```python
from build123d import *

# Parameters (mm, degrees)
F1_DEPTH = 88.9
F2_START = 25.4
F2_DEPTH = 19.05


with BuildPart() as f1:
    # F0 (on Front) → F1 (new body)
    with BuildSketch(Plane.XZ):
        Polygon((-284.0362622675, 569.4989632036), (-303.0862622675, 588.5489632036), (-303.0862622675, -313.1510367964), (-284.0362622675, -294.1010367964), align=None)
        Polygon((243.0137377325, 588.5489632036), (-303.0862622675, 588.5489632036), (-284.0362622675, 569.4989632036), (223.9637377325, 569.4989632036), align=None)
        Polygon((-284.0362622675, -294.1010367964), (-303.0862622675, -313.1510367964), (243.0137377325, -313.1510367964), (223.9637377325, -294.1010367964), align=None)
        Polygon((243.0137377325, -313.1510367964), (243.0137377325, 588.5489632036), (223.9637377325, 569.4989632036), (223.9637377325, -294.1010367964), align=None)
    extrude(amount=F1_DEPTH)

    # F0 (on Front) → F2 (join)
    with BuildSketch(Plane.XZ.offset(F2_START)):
        Polygon((223.9637377325, 569.4989632036), (-284.0362622675, 569.4989632036), (-245.9362622675, 531.3989632036), (185.8637377325, 531.3989632036), align=None)
        Polygon((-245.9362622675, 531.3989632036), (-284.0362622675, 569.4989632036), (-284.0362622675, -294.1010367964), (-245.9362622675, -256.0010367964), align=None)
        Polygon((223.9637377325, -294.1010367964), (223.9637377325, 569.4989632036), (185.8637377325, 531.3989632036), (185.8637377325, -256.0010367964), align=None)
        Polygon((-245.9362622675, -256.0010367964), (-284.0362622675, -294.1010367964), (223.9637377325, -294.1010367964), (185.8637377325, -256.0010367964), align=None)
    extrude(amount=F2_DEPTH)


solid = f1.part
```
Model file for the job. Use its own axes, mm. A direction names the side the tool comes from. Coordinates: 2 decimals unless noted, no trailing zeros. Order: outer loops, then holes, each group sorted by start corner. A loop starts at its lowest first (then second) coordinate and runs counter-clockwise, first axis right, second up. Notation, with made-up numbers: (49.25, -36.75) -> (80.25, -36.75) arc R30 ccw to (80.25, 2.25) -> close; hole circle Ø6 at (51, -33). An arc over 180 degrees is marked (long way). Return JSON: item names as keys, results as strings.
Item 1: Slice it at B-B (z = -153). Write the cut outline in (x, y).
Model answer:
{"outline": "(-303.09, -88.9) -> (-284.04, -88.9) -> (-284.04, -44.45) -> (-245.94, -44.45) -> (-245.94, -25.4) -> (-284.04, -25.4) -> (-284.04, 0) -> (-303.09, 0) -> close; (185.86, -44.45) -> (223.96, -44.45) -> (223.96, -88.9) -> (243.01, -88.9) -> (243.01, 0) -> (223.96, 0) -> (223.96, -25.4) -> (185.86, -25.4) -> close"}
Item 2: 3-axis set-ups, long thin cutter, end or side, ignore diameter. For faces 1 (the face through (-257, -44.45, 172)), 2 (the face through (-245.936, -35, 132)), 3 (the face through (-34, -13, 569.499)), 4 (the face through (-294, -88.9, 140)): which of +Z, -Z, +X, -X, +Y, -Y reach the whole face in a straight line?
Model answer:
{"face 1": "-Y", "face 2": "+Y, -Y", "face 3": "+Y", "face 4": "+Z, -Z, +X, -X, -Y"}
Item 3: Slice it at A-A (x = 65). Write the cut outline in (y, z), then the cut area to 3 significant figures.
Model answer:
{"outline": "(-88.9, -313.15) -> (0, -313.15) -> (0, -294.1) -> (-25.4, -294.1) -> (-25.4, -256) -> (-44.45, -256) -> (-44.45, -294.1) -> (-88.9, -294.1) -> close; (-88.9, 569.5) -> (-44.45, 569.5) -> (-44.45, 531.4) -> (-25.4, 531.4) -> (-25.4, 569.5) -> (0, 569.5) -> (0, 588.55) -> (-88.9, 588.55) -> close", "area": "4,840 mm²"}
Item 4: Mould opens along X. For faces 5 (the face through (-34, -44, -313.151)), 6 (the face through (-303.086, -44, 144)), 7 (the face through (223.964, -66, 144)) say: pulls with the +X half, pulls with the -X half, needs draft (parallel to the pull), parting line crosses it, or undercut.
Model answer:
{"face 5": "needs draft", "face 6": "pulls with the -X half", "face 7": "undercut"}
Item 5: Wall check: line 1 along X through (y, z) = (-65, 450); line 2 along Z through (x, y) = (55, -81.5); line 3 along Z through (x, y) = (54.5, -39.5). Give the ranges that are in metal, low to high. Write a range as from..to.
Model answer:
{"line 1": "x = -303.09..-284.04, 223.96..243.01", "line 2": "z = -313.15..-294.1, 569.5..588.55", "line 3": "z = -313.15..-256, 531.4..588.55"}
Item 6: Slice it at C-C (y = -61). Write the cut outline in (x, z).
Model answer:
{"outline": "(-303.09, -313.15) -> (243.01, -313.15) -> (243.01, 588.55) -> (-303.09, 588.55) -> close; hole (-284.04, -294.1) -> (223.96, -294.1) -> (223.96, 569.5) -> (-284.04, 569.5) -> close"}
